Read the model definition and answer for the solid it produces. Units are mm, in the model's axes. Face numbers are marked on the shaded views. A direction names the side the tool comes from. Round coordinates to 2 decimals unless told otherwise and drop trailing zeros. Order: outer loops, then holes, each group sorted by start corner. A loop starts at its lowest first (then second) coordinate and runs counter-clockwise, first axis right, second up. Notation, with made-up numbers: (83, 52) -> (139, 52) arc R10 ccw to (139, 60) -> close; hole circle Ø4 at (3, -27.75). An arc over 180 degrees is marked (long way). Answer as a JSON object with one key per item and string values. Group by question number.
Item 1: Consider probe 1 along Z at (x, y) = (-0.5, 91); probe 2 along X at (y, z) = (105, -41.5); probe 3 along X at (y, z) = (-3.5, -36.5) (3 decimals). Determine where each line is inside the solid, lowest interval first. Write a range as from..to.
Item 2: Section B-B, the plane x = -31.5 is taken. Write down the section's boundary in (y, z), plus the area to 3 significant figures.
Item 3: The mould has two halves that part along X. Classify the marked faces 6, 7 and 8: pulls with the +X half, pulls with the -X half, needs draft (parallel to the pull), parting line crosses it, or undercut.
Item 4: Given P1, Ø8.5, axis at y = -3.5, z = 36, coming from the -X side (3 decimals); P2, Ø2, axis at x = 4, z = -0.5, coming from the -Y side; P3, Ø11.5, axis at y = 82, z = -2.5, coming from the -X side, each flat-ended and moving along its own axis, determine where each tip first touches the part or whether it passes through.
Item 5: Section A-A, the plane z = -7.5 is taken. Count the separate pieces of the cut face and the enclosed holes in it, plus the area to 3 significant figures.
Item 6: For the marked faces 1, 2, 3, 4 and 5, determine the directions among +Z, -Z, +X, -X, +Y, -Y from which every point of the face is accessible in a straight line to the end or side of a thin tool.
Item 7: Section C-C, the plane y = 34.5 is taken. Write down the section's boundary in (x, z).
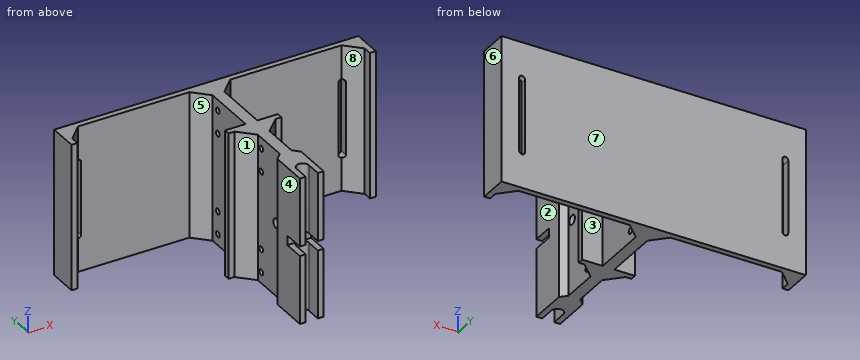
from build123d import *

# Parameters (mm, degrees)
F2_DEPTH     = 50
F3_T1_DEPTH  = 100
F3_T6_DEPTH  = 100
F3_T11_DEPTH = 100
F5_R         = 2
F6_DEPTH     = 8
F8_DEPTH     = 6.001
F9_R         = 3.25
F10_DEPTH    = 25


# Not quite as in the source:
# - a fillet or chamfer that OpenCascade refuses, or shapes differently, is made with other operations: its cross-section is extruded or revolved along the edge and cut away or added


with BuildPart() as f2:
    # F1 (on Top) → F2 (new body, symmetric)
    with BuildSketch(Plane.XY):
        with BuildLine():
            Line((-8.125, 9.6056647934), (-8.125, -10.3943352066))
            Line((-8.125, -10.3943352066), (-4.125, -10.3943352066))
            Line((-4.125, -10.3943352066), (-4.125, 0))
            ThreePointArc((-4.125, 0), (0, 4.125), (4.125, 0))
            Line((4.125, 0), (4.125, -10.3943352066))
            Line((4.125, -10.3943352066), (8.125, -10.3943352066))
            Line((8.125, -10.3943352066), (8.125, 9.6056647934))
            Line((8.125, 9.6056647934), (4, 9.6056647934))
            Line((4, 9.6056647934), (4, 55))
            Line((4, 55), (18, 55))
            Line((18, 55), (18, 59))
            Line((18, 59), (4, 59))
            Line((4, 59), (4, 107))
            Line((4, 107), (100, 107))
            Line((100, 107), (100, 91))
            Line((100, 91), (104, 91))
            Line((104, 91), (104, 111))
            Line((104, 111), (0, 111))
            Line((0, 111), (-104, 111))
            Line((-104, 111), (-104, 91))
            Line((-104, 91), (-100, 91))
            Line((-100, 91), (-100, 107))
            Line((-100, 107), (-4, 107))
            Line((-4, 107), (-4, 59))
            Line((-4, 59), (-18, 59))
            Line((-18, 59), (-18, 55))
            Line((-18, 55), (-4, 55))
            Line((-4, 55), (-4, 9.6056647934))
            Line((-4, 9.6056647934), (-8.125, 9.6056647934))
        make_face()
    extrude(amount=F2_DEPTH, both=True)

    # F3: chamfer of 10 on 8 edges, made by hand

    # F3_s2 → F3_t1 (join)
    with BuildSketch(Plane.XY.offset(-50)):
        Polygon((14, 55), (4, 45), (4, 55), align=None)
        Polygon((-4, 45), (-14, 55), (-4, 55), align=None)
        Polygon((14, 107), (4, 97), (4, 107), align=None)
        Polygon((-4, 97), (-14, 107), (-4, 107), align=None)
        Polygon((100, 97), (90, 107), (100, 107), align=None)
        Polygon((-90, 107), (-100, 97), (-100, 107), align=None)
    extrude(amount=F3_T1_DEPTH)


with BuildPart() as f3_tool4:
    # F3_s5 → F3_t6 (new body)
    with BuildSketch(Plane.XY.offset(-50)):
        Polygon((4, 19.6056647934), (14, 9.6056647934), (4, 9.6056647934), align=None)
    extrude(amount=F3_T6_DEPTH)

    split(bisect_by=Plane.YZ.offset(8.125), keep=Keep.BOTTOM)


with BuildPart() as f2_1:
    add(f2.part)

    # F3_t3: union F3_tool4
    add(f3_tool4.part)


with BuildPart() as f3_tool9:
    # F3_s10 → F3_t11 (new body)
    with BuildSketch(Plane.XY.offset(50)):
        Polygon((-14, 9.6056647934), (-4, 19.6056647934), (-4, 9.6056647934), align=None)
    extrude(amount=-F3_T11_DEPTH)

    split(bisect_by=Plane.YZ.offset(-8.125), keep=Keep.TOP)


with BuildPart() as f2_2:
    add(f2_1.part)

    # F3_t8: union F3_tool9
    add(f3_tool9.part)

    # F5 (on face) → F6 (cut, through all)
    with BuildSketch(Plane(origin=(-4, 0, 0), x_dir=(0, -1, 0), z_dir=(-1, 0, 0))):
        with Locations((-91, -26.75)):
            Circle(F5_R)
        with Locations((-91, -42.5)):
            Circle(F5_R)
        with Locations((-41, -26.75)):
            Circle(F5_R)
        with Locations((-41, -42.5)):
            Circle(F5_R)
        with Locations((-41, 26.75)):
            Circle(F5_R)
        with Locations((-41, 42.5)):
            Circle(F5_R)
        with Locations((-91, 42.5)):
            Circle(F5_R)
        with Locations((-91, 26.75)):
            Circle(F5_R)
    extrude(amount=-F6_DEPTH, mode=Mode.SUBTRACT)

    # F7 (on face) → F8 (cut, through all)
    with BuildSketch(Plane(origin=(0, 111, 0), x_dir=(-1, 0, 0), z_dir=(0, 1, 0))):
        with BuildLine():
            Line((-91.9984134228, 0), (-91.9984134228, -24.9203520777))
            ThreePointArc((-91.9984134228, -24.9203520777), (-89.9790038693, -26.9998897876), (-88.003699271, -24.8784129963))
            Line((-88.003699271, -24.8784129963), (-88.003699271, 0))
            Line((-88.003699271, 0), (-88.003699271, 24.8784129963))
            ThreePointArc((-88.003699271, 24.8784129963), (-89.9790038693, 26.9998897876), (-91.9984134228, 24.9203520777))
            Line((-91.9984134228, 24.9203520777), (-91.9984134228, 0))
        make_face()
        with BuildLine():
            Line((88.003699271, 0), (88.003699271, -24.8784129963))
            ThreePointArc((88.003699271, -24.8784129963), (89.9790038693, -26.9998897876), (91.9984134228, -24.9203520777))
            Line((91.9984134228, -24.9203520777), (91.9984134228, 0))
            Line((91.9984134228, 0), (91.9984134228, 24.9203520777))
            ThreePointArc((91.9984134228, 24.9203520777), (89.9790038693, 26.9998897876), (88.003699271, 24.8784129963))
            Line((88.003699271, 24.8784129963), (88.003699271, 0))
        make_face()
    extrude(amount=-F8_DEPTH, mode=Mode.SUBTRACT)

    # F9 (on face) → F10 (cut)
    with BuildSketch(Plane.YZ.offset(8.125)):
        Polygon((4, 3.25), (-10.3943352066, 3.25), (-10.3943352066, 0), (-10.3943352066, -3.25), (4, -3.25), (4, 0), align=None)
        with Locations((23.8227438553, 0)):
            Circle(F9_R)
    extrude(amount=-F10_DEPTH, mode=Mode.SUBTRACT)


solid = f2_2.part
Values found:
{
 "1": {"probe 1": "-50..-44.5, -40.5..-28.75, -24.75..24.75, 28.75..40.5, 44.5..50", "probe 2": "-104..-92, -12..12, 92..104", "probe 3": "-8.125..-4.125, 4.125..8.125"},
 "2": {"outline": "(107, -50) -> (111, -50) -> (111, 50) -> (107, 50) -> close", "area": "400 mm2"},
 "3": {"face 6": "pulls with the +X half", "face 7": "needs draft", "face 8": "undercut"},
 "4": {"P1": "x = -8.125", "P2": "y = 4", "P3": "x = -4"},
 "5": {"separate pieces": "3", "enclosed holes": "0", "area": "2,390 mm2"},
 "6": {"face 1": "+Z, -Z, -X", "face 2": "+Z, -Z, +X, -Y", "face 3": "+Z, -Z, +X", "face 4": "+Z, -Z, -X, -Y", "face 5": "+Z, -Z"},
 "7": {"outline": "(-4, -50) -> (4, -50) -> (4, 50) -> (-4, 50) -> close"}
}
